The figure shows three views and two pictorial views of one solid part (mm, origin at its lowest corner). Answer the questions. A direction names the side the tool comes from. Round coordinates to 2 decimals unless told otherwise and drop trailing zeros. Write each loop counter-clockwise with the first axis right and the second up, starting at its lowest first coordinate (ties: lowest second). Pieces come first, ordered by that corner, then holes.
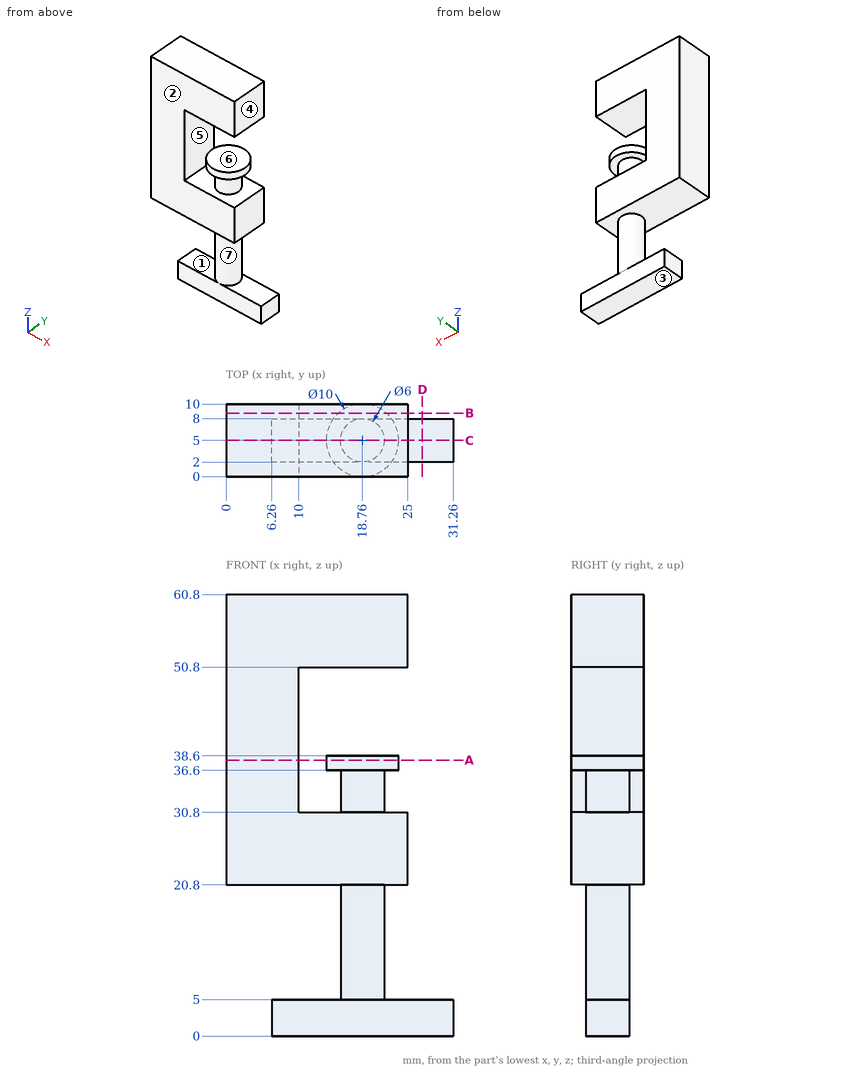
Q1. Section C-C (y = 5) is taken. Determine the outline of the cut face in (x, z).
Verdict:
outline: (0, 20.8) - (15.76, 20.8) - (15.76, 5) - (6.26, 5) - (6.26, 0) - (31.26, 0) - (31.26, 5) - (21.76, 5) - (21.76, 20.8) - (25, 20.8) - (25, 30.8) - (21.76, 30.8) - (21.76, 36.6) - (23.76, 36.6) - (23.76, 38.6) - (13.76, 38.6) - (13.76, 36.6) - (15.76, 36.6) - (15.76, 30.8) - (10, 30.8) - (10, 50.8) - (25, 50.8) - (25, 60.8) - (0, 60.8) - close
Q2. Determine the mould class of the marked faces 1, 2 and 3 for opening direction Z: pulls with the +Z half, pulls with the -Z half, needs draft (parallel to the pull), parting line crosses it, or undercut.
Verdict:
face 1: undercut
face 2: needs draft
face 3: pulls with the -Z half
Q3. Section B-B (y = 8.75) is taken. Determine the outline of the cut face in (x, z).
Verdict:
outline: (0, 20.8) - (25, 20.8) - (25, 30.8) - (10, 30.8) - (10, 50.8) - (25, 50.8) - (25, 60.8) - (0, 60.8) - close; (15.45, 36.6) - (22.07, 36.6) - (22.07, 38.6) - (15.45, 38.6) - close
Q4. Section D-D (x = 27) is taken. Determine the outline of the cut face in (y, z), then the cut area to 3 significant figures.
Verdict:
outline: (2, 0) - (8, 0) - (8, 5) - (2, 5) - close
area: 30.0 mm2
Q5. Flat-ended cylindrical pins translate along their axes: pin 1 Ø5 at (y, z) = (7, 38.5) entering from +X; pin 2 Ø4 at (x, z) = (17, 3) entering from -Y; pin 3 Ø5.5 at (x, z) = (13.5, 3) entering from +Y. Find the tip coordinate at first contact, or state that the pin passes through.
Verdict:
pin 1: stops at x = 23.76
pin 2: stops at y = 2
pin 3: stops at y = 8
Q6. Straight lines are drawn through the part: probe 1 along Z at (x, y) = (23.5, 7.5); probe 2 along Z at (x, y) = (24.5, 8.5); probe 3 along X at (y, z) = (5, 33). For each, find the intervals that lie inside material, in ascending order.
Verdict:
probe 1: z = 0 to 5, 20.8 to 30.8, 50.8 to 60.8
probe 2: z = 20.8 to 30.8, 50.8 to 60.8
probe 3: x = 0 to 10, 15.76 to 21.76
Q7. Section A-A (z = 38) is taken. Determine the outline of the cut face in (x, y).
Verdict:
outline: (0, 0) - (10, 0) - (10, 10) - (0, 10) - close; circle Ø10 at (18.76, 5)
Q8. Which of the six approach directions +Z, -Z, +X, -X, +Y, -Y give full straight-line access (tool end or side, diameter ignored) to the marked faces 4, 5, 6 and 7?
Verdict:
face 4: +Z, +X, +Y, -Y
face 5: +Y, -Y
face 6: +X, +Y, -Y
face 7: none
